from build123d import *

# Parameters (mm, degrees)
F1_DEPTH = 1.905


with BuildPart() as f1:
    # F0 (on Top) → F1 (new body)
    with BuildSketch(Plane.XY):
        with BuildLine():
            Line((-4.878408, 6.86215), (-3.837505, 5.059254))
            ThreePointArc((-3.837505, 5.059254), (-5.499261, 3.175), (-6.300195, 0.79375))
            Line((-6.300195, 0.79375), (-8.382, 0.79375))
            Line((-8.382, 0.79375), (-8.382, -0.79375))
            Line((-8.382, -0.79375), (-6.300195, -0.79375))
            ThreePointArc((-6.300195, -0.79375), (-5.499261, -3.175), (-3.837505, -5.059254))
            Line((-3.837505, -5.059254), (-4.878408, -6.86215))
            Line((-4.878408, -6.86215), (-3.503592, -7.6559))
            Line((-3.503592, -7.6559), (-2.46269, -5.853004))
            ThreePointArc((-2.46269, -5.853004), (0, -6.35), (2.46269, -5.853004))
            Line((2.46269, -5.853004), (3.503592, -7.6559))
            Line((3.503592, -7.6559), (4.878408, -6.86215))
            Line((4.878408, -6.86215), (3.837505, -5.059254))
            ThreePointArc((3.837505, -5.059254), (5.499261, -3.175), (6.300195, -0.79375))
            Line((6.300195, -0.79375), (8.382, -0.79375))
            Line((8.382, -0.79375), (8.382, 0.79375))
            Line((8.382, 0.79375), (6.300195, 0.79375))
            ThreePointArc((6.300195, 0.79375), (5.499261, 3.175), (3.837505, 5.059254))
            Line((3.837505, 5.059254), (4.878408, 6.86215))
            Line((4.878408, 6.86215), (3.503592, 7.6559))
            Line((3.503592, 7.6559), (2.46269, 5.853004))
            ThreePointArc((2.46269, 5.853004), (0, 6.35), (-2.46269, 5.853004))
            Line((-2.46269, 5.853004), (-3.503592, 7.6559))
            Line((-3.503592, 7.6559), (-4.878408, 6.86215))
        make_face()
        with BuildLine():
            ThreePointArc((-3.19621, -3.948498), (-4.399409, -2.54), (-5.017605, -0.79375))
            Line((-5.017605, -0.79375), (-3.726401, -0.79375))
            ThreePointArc((-3.726401, -0.79375), (-3.299557, -1.905), (-2.550608, -2.830283))
            Line((-2.550608, -2.830283), (-3.19621, -3.948498))
        make_face(mode=Mode.SUBTRACT)
        with BuildLine():
            ThreePointArc((1.821395, -4.742248), (0, -5.08), (-1.821395, -4.742248))
            Line((-1.821395, -4.742248), (-1.175793, -3.624033))
            ThreePointArc((-1.175793, -3.624033), (0, -3.81), (1.175793, -3.624033))
            Line((1.175793, -3.624033), (1.821395, -4.742248))
        make_face(mode=Mode.SUBTRACT)
        with BuildLine():
            Line((3.726401, -0.79375), (5.017605, -0.79375))
            ThreePointArc((5.017605, -0.79375), (4.399409, -2.54), (3.19621, -3.948498))
            Line((3.19621, -3.948498), (2.550608, -2.830283))
            ThreePointArc((2.550608, -2.830283), (3.299557, -1.905), (3.726401, -0.79375))
        make_face(mode=Mode.SUBTRACT)
        with BuildLine():
            ThreePointArc((-5.017605, 0.79375), (-4.399409, 2.54), (-3.19621, 3.948498))
            Line((-3.19621, 3.948498), (-2.550608, 2.830283))
            ThreePointArc((-2.550608, 2.830283), (-3.299557, 1.905), (-3.726401, 0.79375))
            Line((-3.726401, 0.79375), (-5.017605, 0.79375))
        make_face(mode=Mode.SUBTRACT)
        with BuildLine():
            ThreePointArc((-2.412791, 0.79375), (-2.199705, 1.27), (-1.893803, 1.692663))
            Line((-1.893803, 1.692663), (-1.482902, 0.980962))
            ThreePointArc((-1.482902, 0.980962), (-0.889, 1.539793), (-0.108087, 1.774712))
            Line((-0.108087, 1.774712), (-0.518988, 2.486413))
            ThreePointArc((-0.518988, 2.486413), (0, 2.54), (0.518988, 2.486413))
            Line((0.518988, 2.486413), (0.108087, 1.774712))
            ThreePointArc((0.108087, 1.774712), (0.889, 1.539793), (1.482902, 0.980962))
            Line((1.482902, 0.980962), (1.893803, 1.692663))
            ThreePointArc((1.893803, 1.692663), (2.199705, 1.27), (2.412791, 0.79375))
            Line((2.412791, 0.79375), (1.590989, 0.79375))
            ThreePointArc((1.590989, 0.79375), (1.778, 0), (1.590989, -0.79375))
            Line((1.590989, -0.79375), (2.412791, -0.79375))
            ThreePointArc((2.412791, -0.79375), (2.199705, -1.27), (1.893803, -1.692663))
            Line((1.893803, -1.692663), (1.482902, -0.980962))
            ThreePointArc((1.482902, -0.980962), (0.889, -1.539793), (0.108087, -1.774712))
            Line((0.108087, -1.774712), (0.518988, -2.486413))
            ThreePointArc((0.518988, -2.486413), (0, -2.54), (-0.518988, -2.486413))
            Line((-0.518988, -2.486413), (-0.108087, -1.774712))
            ThreePointArc((-0.108087, -1.774712), (-0.889, -1.539793), (-1.482902, -0.980962))
            Line((-1.482902, -0.980962), (-1.893803, -1.692663))
            ThreePointArc((-1.893803, -1.692663), (-2.199705, -1.27), (-2.412791, -0.79375))
            Line((-2.412791, -0.79375), (-1.590989, -0.79375))
            ThreePointArc((-1.590989, -0.79375), (-1.778, 0), (-1.590989, 0.79375))
            Line((-1.590989, 0.79375), (-2.412791, 0.79375))
        make_face(mode=Mode.SUBTRACT)
        with BuildLine():
            ThreePointArc((3.19621, 3.948498), (4.399409, 2.54), (5.017605, 0.79375))
            Line((5.017605, 0.79375), (3.726401, 0.79375))
            ThreePointArc((3.726401, 0.79375), (3.299557, 1.905), (2.550608, 2.830283))
            Line((2.550608, 2.830283), (3.19621, 3.948498))
        make_face(mode=Mode.SUBTRACT)
        with BuildLine():
            Line((-1.175793, 3.624033), (-1.821395, 4.742248))
            ThreePointArc((-1.821395, 4.742248), (0, 5.08), (1.821395, 4.742248))
            Line((1.821395, 4.742248), (1.175793, 3.624033))
            ThreePointArc((1.175793, 3.624033), (0, 3.81), (-1.175793, 3.624033))
        make_face(mode=Mode.SUBTRACT)
    extrude(amount=F1_DEPTH)


solid = f1.part
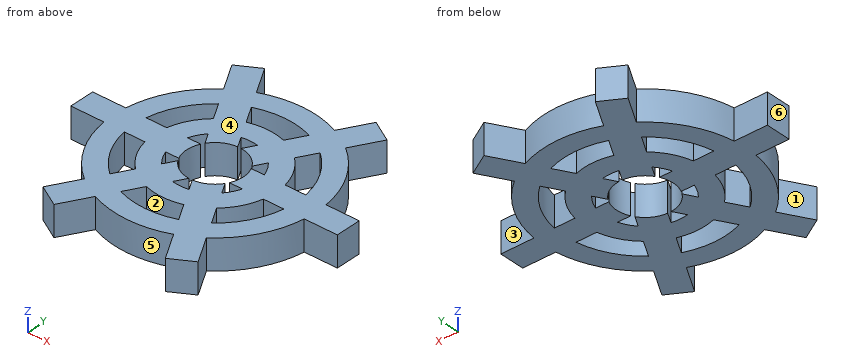
Check sheet for the modelled part. Datum: model origin and axes. Units: mm. Face numbers are marked on the shaded views. A direction names the side the tool comes from. Round coordinates to 2 decimals unless told otherwise and drop trailing zeros. Order: outer loops, then holes, each group sorted by start corner. A loop starts at its lowest first (then second) coordinate and runs counter-clockwise, first axis right, second up. Notation, with made-up numbers: M 40,70.5 L 68,70.5 A25 cw 68,91.5 Z; hole C 24.5,-17 d7. An arc over 180 degrees is marked long. One line per item, written item: value. Start each with the question number.
1. Gauge pin test, flat ends, axial feed: P1, Ø1, axis at x = -4.5, z = 1, coming from the +Y side; P2, Ø0.7, axis at x = 2, z = 0.5, coming from the +Y side; P3, Ø0.6, axis at x = 7, z = 1, coming from the +Y side. Record the tip position at first contact, or that the pin passes through.
2. Scan lines: line 1 along Y through (x, z) = (-1, 1.25); line 2 along X through (y, z) = (3, 1.1); line 3 along Y through (x, z) = (-0.75, 0.35). Record each from-to range of solid material in increasing order.
3. Release check for a two-part mould opening along X. For the marked faces 4, 5 and 6 record: released by +X, released by -X, zero draft, split by the parting line, or undercut.
4. Section check A-A on y = -1.25. Enter the section's corners in (x, z) (3 decimals), and give its area (3 significant figures).
5. Section check B-B on x = 3. Enter the section's corners in (y, z) (3 decimals), and give its area (3 significant figures).
6. Access from +Z, -Z, +X, -X, +Y, -Y to the whole of each face (thin tool, end or side, straight path). Record for the marked faces 1, 2 and 3.
7. Section check C-C on y = 4.25. Enter the section's corners in (x, z) (3 decimals), and give its area (3 significant figures).
8. Section check D-D on z = 1.35. Give the number of separate pieces and of enclosed holes in the cut face, and give its area (3 significant figures).
Results found:
1. P1: y = 7.37
1. P2: y = 6.13
1. P3: y = 0.79
2. line 1: -6.27 to -4.98, -3.68 to -1.47, 1.47 to 3.68, 4.98 to 6.27
2. line 2: -5.6 to -4.1, -2.65 to 2.65, 4.1 to 5.6
2. line 3: -6.31 to -5.02, -3.74 to -1.61, 1.61 to 3.74, 5.02 to 6.31
3. face 4: zero draft
3. face 5: undercut
3. face 6: released by -X
4. outline: M -6.226,0 L -4.924,0 L -4.924,1.905 L -6.226,1.905 Z; M -3.599,0 L -2.211,0 L -2.211,1.905 L -3.599,1.905 Z; M -1.638,0 L -1.264,0 L -1.264,1.905 L -1.638,1.905 Z; M 1.264,0 L 1.638,0 L 1.638,1.905 L 1.264,1.905 Z; M 2.211,0 L 3.599,0 L 3.599,1.905 L 2.211,1.905 Z; M 4.924,0 L 6.226,0 L 6.226,1.905 L 4.924,1.905 Z
4. area: 11.7 mm^2
5. outline: M -6.784,0 L -3.609,0 L -3.609,1.905 L -6.784,1.905 Z; M -2.349,0 L 2.349,0 L 2.349,1.905 L -2.349,1.905 Z; M 3.609,0 L 6.784,0 L 6.784,1.905 L 3.609,1.905 Z
5. area: 21.0 mm^2
6. face 1: +Z, -Z, -X
6. face 2: +Z, -Z
6. face 3: +Z, -Z, +X, +Y
7. outline: M -4.718,0 L -1.537,0 L -1.537,1.905 L -4.718,1.905 Z; M 1.537,0 L 4.718,0 L 4.718,1.905 L 1.537,1.905 Z
7. area: 12.1 mm^2
8. separate pieces: 1
8. enclosed holes: 7
8. area: 110 mm^2
